from build123d import *

# Parameters (mm, degrees)
SKETCH1_R           = 76.2
BOSS_EXTRUDE1_DEPTH = 3.175
SKETCH2_R           = 25.4
CUT_EXTRUDE1_DEPTH  = 3.175
SKETCH3_R           = 6.35
CUT_EXTRUDE2_DEPTH  = 10


with BuildPart() as part:
    # Sketch1 → Boss-Extrude1 (new body)
    with BuildSketch(Plane(origin=(0, 0, 0), x_dir=(1, 0, 0), z_dir=(0, 1, 0))):
        with Locations(Location((0, 0, 0), (0, 0, 270))):
            Circle(SKETCH1_R)
        Polygon((-50, 50), (-50, 44), (-51.5875, 44), (-51.5875, 51.5875), (-44, 51.5875), (-44, 50), align=None, mode=Mode.SUBTRACT)
        Polygon((51.5875, -44), (50, -44), (50, -50), (44, -50), (44, -51.5875), (51.5875, -51.5875), align=None, mode=Mode.SUBTRACT)
        Polygon((-50, -50), (-44, -50), (-44, -51.5875), (-51.5875, -51.5875), (-51.5875, -44), (-50, -44), align=None, mode=Mode.SUBTRACT)
        Polygon((51.5875, 51.5875), (44, 51.5875), (44, 50), (50, 50), (50, 44), (51.5875, 44), align=None, mode=Mode.SUBTRACT)
    extrude(amount=BOSS_EXTRUDE1_DEPTH)

    # Sketch2 → Cut-Extrude1 (cut)
    with BuildSketch(Plane(origin=(0, 3.175, 0), x_dir=(1, 0, 0), z_dir=(0, 1, 0))):
        with Locations(Location((0, 0, 0), (0, 0, 270))):
            Circle(SKETCH2_R)
    extrude(amount=-CUT_EXTRUDE1_DEPTH, mode=Mode.SUBTRACT)

    # Sketch3 → Cut-Extrude2 (cut)
    with BuildSketch(Plane(origin=(0, 3.175, 0), x_dir=(1, 0, 0), z_dir=(0, 1, 0))):
        with Locations(Location((-64.2875, 0, 0), (0, 0, 270))):
            Circle(SKETCH3_R)
        with Locations(Location((64.2875, 0, 0), (0, 0, 270))):
            Circle(SKETCH3_R)
    extrude(amount=-CUT_EXTRUDE2_DEPTH, mode=Mode.SUBTRACT)


solid = part.part
Part model, mm, in its own coordinate system. Coordinates: 2 decimals unless noted, no trailing zeros. Write each loop counter-clockwise with the first axis right and the second up, starting at its lowest first coordinate (ties: lowest second). Pieces come first, ordered by that corner, then holes. Notation, with made-up numbers: (-36.75, 46.5) - (3.25, 46.5) arc R7 cw to (3.25, 57.5) - close; hole circle Ø7 at (-2, 20). An arc over 180 degrees is marked (long way). Put each result on its own line as item: value.
1. Probe line 1 along X through (y, z) = (2.5, 0); line 2 along X through (y, z) = (2.75, 51.5); line 3 along Z through (x, y) = (-50.5, 0.35). List the from-to ranges inside material, lowest first. Write a range as [from, to].
Final values:
line 1: x = [-76.2, -70.64], [-57.94, -25.4], [25.4, 57.94], [70.64, 76.2]
line 2: x = [-56.16, -51.59], [-44, 44], [51.59, 56.16]
line 3: z = [-57.06, -51.59], [-44, 44], [51.59, 57.06]
2. Band-saw the part on C-C (z = -19). Write the cut outline in (x, y) (3 decimals), then the cut area to 3 significant figures.
Final values:
outline: (-73.793, 0) - (-16.857, 0) - (-16.857, 3.175) - (-73.793, 3.175) - close; (16.857, 0) - (73.793, 0) - (73.793, 3.175) - (16.857, 3.175) - close
area: 362 mm²
3. Band-saw the part on D-D (y = 2). Write the cut outline in (x, z).
Final values:
outline: circle Ø152.4 at (0, 0); hole circle Ø12.7 at (-64.29, 0); hole (-51.59, -51.59) - (-44, -51.59) - (-44, -50) - (-50, -50) - (-50, -44) - (-51.59, -44) - close; hole (-51.59, 44) - (-50, 44) - (-50, 50) - (-44, 50) - (-44, 51.59) - (-51.59, 51.59) - close; hole circle Ø50.8 at (0, 0); hole (44, -51.59) - (51.59, -51.59) - (51.59, -44) - (50, -44) - (50, -50) - (44, -50) - close; hole (44, 50) - (50, 50) - (50, 44) - (51.59, 44) - (51.59, 51.59) - (44, 51.59) - close; hole circle Ø12.7 at (64.29, 0)
4. Band-saw the part on A-A (z = 0). Write the cut outline in (x, y) (1 decimal), then the cut area to 3 significant figures.
Final values:
outline: (-76.2, 0) - (-70.6, 0) - (-70.6, 3.2) - (-76.2, 3.2) - close; (-57.9, 0) - (-25.4, 0) - (-25.4, 3.2) - (-57.9, 3.2) - close; (25.4, 0) - (57.9, 0) - (57.9, 3.2) - (25.4, 3.2) - close; (70.6, 0) - (76.2, 0) - (76.2, 3.2) - (70.6, 3.2) - close
area: 242 mm²
5. Flat gauge pins, fed straight in: pin 1 Ø1.6 at (x, y) = (-46, 1) entering from +Z; pin 2 Ø0.5 at (y, z) = (1, -51) entering from +X; pin 3 Ø0.5 at (x, y) = (-50.5, 1) entering from +Z. Where does each tip first touch, or does it go through?
Final values:
pin 1: stops at z = 61.35
pin 2: stops at x = 56.84
pin 3: stops at z = 57.28
6. Band-saw the part on B-B (x = 0). Write the cut outline in (y, z) (3 decimals).
Final values:
outline: (0, -76.2) - (3.175, -76.2) - (3.175, -25.4) - (0, -25.4) - close; (0, 25.4) - (3.175, 25.4) - (3.175, 76.2) - (0, 76.2) - close
